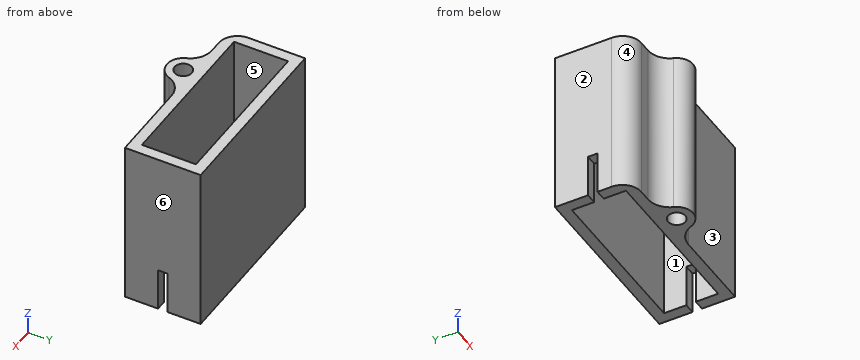
Autodesk Inventor part; units mm, degrees
ref_plane "YZ Plane" through (0, 0, 0) normal (1, 0, 0) x (0, 1, 0)
ref_plane "XZ Plane" through (0, 0, 0) normal (0, 1, 0) x (-1, 0, 0)
ref_plane "XY Plane" through (0, 0, 0) normal (0, 0, 1) x (1, 0, 0)
sketch "Sketch1" plane through (0, 0, 0) normal (0, 0, 1) x (1, 0, 0)
  line L0 (-15, -5) -> (15, -5)
  line L1 (15, -5) -> (15, 5)
  line L2 (15, 5) -> (-15, 5)
  line L3 (-15, 5) -> (-15, -5)
  line L4 (-15, -5) -> (15, 5) construction
  line L5 (15, -5) -> (-15, 5) construction
  line L6 (-17, 7) -> (17, 7)
  line L7 (17, 7) -> (17, -7)
  line L8 (17, -7) -> (-17, -7)
  line L9 (-17, -7) -> (-17, 7)
  line L10 (-15, 0) -> (-8.5, 0) construction
  line L11 (-8.5, 0) -> (-4.7776, -8.5875) construction
  circle A0 centre (-13.2482, 10.9542) radius 1.5875
  circle A1 centre (-13.2482, 10.9542) radius 3
  line L12 (-13.2482, 10.9542) -> (-19.3708, 3.6576) construction
  line L13 (-19.3708, 3.6576) -> (-4.7776, -8.5875) construction
  circle A2 centre (-4.7776, -8.5875) radius 1.5875
  circle A3 centre (-4.7776, -8.5875) radius 3
  point P0 (0, 0)
  point P1 (-2.2321, -7)
  point P2 (-9.2647, 7)
  point P3 (-13.8861, 7)
  point P4 (-7.3232, -7)
  dimension "d0" = 10
  dimension "d1" = 30
  dimension "d2" = 2
  dimension "d3" = 6.5
  dimension "d8" = 3.175
  dimension "d9" = 6
  dimension "d10" = 9.525
  dimension "d11" = 19.05
  dimension "d12" = 3.175
  dimension "d13" = 6
  dimension "d14" = 40
extrude "Extrusion1" add sketch "Sketch1" along normal blind 31 contours L6 L7 L8 A3 L9 | A3 L8 | L8 A3
fillet "Fillet1" radius 4 2 edges at (-2.2321, -7, 15.5) (-7.3232, -7, 15.5)
sketch "Sketch2" plane through (0, 0, 0) normal (0, 0, -1) x (-1, 0, 0)
  line L0 (-22.5, -0.875) -> (22.5, -0.875)
  line L1 (22.5, -0.875) -> (22.5, 0.875)
  line L2 (22.5, 0.875) -> (-22.5, 0.875)
  line L3 (-22.5, 0.875) -> (-22.5, -0.875)
  line L4 (-22.5, -0.875) -> (22.5, 0.875) construction
  line L5 (22.5, -0.875) -> (-22.5, 0.875) construction
  point P0 (0, 0)
  dimension "d18" = 45
  dimension "d19" = 1.75
extrude "Extrusion2" cut sketch "Sketch2" against normal blind 8
fillet "Fillet2" radius 3.5 1 edges at (-17, -7, 15.5)
properties part number "Sleeve" material "Nylon 6/6"
Part model, mm, in its own coordinate system. Face numbers are marked on the shaded views. A direction names the side the tool comes from. Coordinates: 2 decimals unless noted, no trailing zeros. Order: outer loops, then holes, each group sorted by start corner. A loop starts at its lowest first (then second) coordinate and runs counter-clockwise, first axis right, second up. Notation, with made-up numbers: (68.5, -13) -> (88.5, -13) arc R19 ccw to (88.5, 20) -> close; hole circle Ø7 at (45.5, -36.5). An arc over 180 degrees is marked (long way). Put each result on its own line as item: value. Start each with the question number.
(1) Band-saw the part on D-D (x = -4.5). Give the cut face in (y, z), then the cut area to 3 significant figures.
(2) Probe line 1 along Y through (x, z) = (14, 20); line 2 along Y through (x, z) = (-4.5, 7); line 3 along X through (y, z) = (-2.25, 23). List the from-to ranges inside material, lowest first. Write a range as [from, to].
(3) Band-saw the part on C-C (z = 5). Give the cut face in (x, y) (1 decimal).
(4) Pin check, flat tips, straight feed: pin 1 Ø0.6 at (x, z) = (16.5, 4) entering from -Y; pin 2 Ø0.9 at (x, y) = (16, -0.5) entering from -Z; pin 3 Ø4 at (x, z) = (3, 26.5) entering from -Y; pin 4 Ø2 at (x, z) = (-15.5, 2.5) entering from -Y. Stop position of each tip, or through.
(5) Mould opens along X. For the marked faces 4, 5 and 6 say: pulls with the +X half, pulls with the -X half, needs draft (parallel to the pull), parting line crosses it, or undercut.
(6) Band-saw the part on B-B (y = 0.25). Give the cut face in (x, z).
(7) Band-saw the part on A-A (x = 9). Give the cut face in (y, z), then the cut area to 3 significant figures.
(8) Which spindle directions (+Z, -Z, +X, -X, +Y, -Y) get a long thin tool onto all of the face, cutting with end or side? Do the marked faces 1, 2 and 3. Say none if no direction does.
Determined:
1. outline: (-11.57, 0) -> (-10.15, 0) -> (-10.15, 31) -> (-11.57, 31) -> close; (-7.02, 0) -> (-5, 0) -> (-5, 31) -> (-7.02, 31) -> close; (5, 0) -> (7, 0) -> (7, 31) -> (5, 31) -> close
1. area: 169 mm²
2. line 1: y = [-7, -5], [5, 7]
2. line 2: y = [-11.57, -10.15], [-7.02, -5], [5, 7]
2. line 3: x = [-17, -15], [15, 17]
3. outline: (-17, -3.5) arc R3.5 ccw to (-13.5, -7) -> (-11.3, -7) arc R4 cw to (-7.6, -9.6) arc R3 ccw to (-2, -9.6) arc R4 cw to (1.8, -7) -> (17, -7) -> (17, -0.9) -> (15, -0.9) -> (15, -5) -> (-15, -5) -> (-15, -0.9) -> (-17, -0.9) -> close; (-17, 0.9) -> (-15, 0.9) -> (-15, 5) -> (15, 5) -> (15, 0.9) -> (17, 0.9) -> (17, 7) -> (-17, 7) -> close; hole circle Ø3.2 at (-4.8, -8.6)
4. pin 1: stops at y = -7
4. pin 2: stops at z = 0
4. pin 3: stops at y = -7.08
4. pin 4: stops at y = -6.85
5. face 4: pulls with the -X half
5. face 5: undercut
5. face 6: pulls with the +X half
6. outline: (-17, 8) -> (-15, 8) -> (-15, 31) -> (-17, 31) -> close; (15, 8) -> (17, 8) -> (17, 31) -> (15, 31) -> close
7. outline: (-7, 0) -> (-5, 0) -> (-5, 31) -> (-7, 31) -> close; (5, 0) -> (7, 0) -> (7, 31) -> (5, 31) -> close
7. area: 124 mm²
8. face 1: +Z, -Z
8. face 2: +Z, -Z, -X, +Y, -Y
8. face 3: +Z, -Z, +X, -Y
